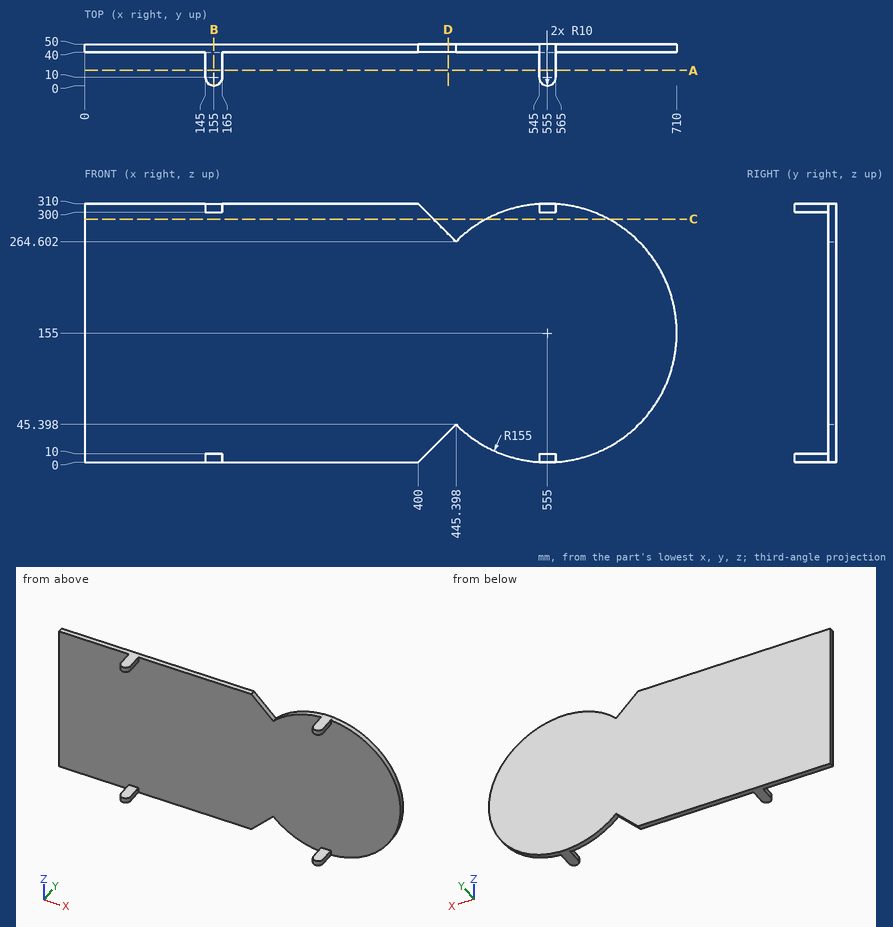
Job drawing, mm, ordinate dimensions from the low corner. One solid piece. Coordinates: 2 decimals unless noted, no trailing zeros. Order: outer loops, then holes, each group sorted by start corner. A loop starts at its lowest first (then second) coordinate and runs counter-clockwise, first axis right, second up. Notation, with made-up numbers: (24, 19) - (29, 19) arc R21 cw to (29, 24) - close; hole circle Ø4 at (31.5, 64). An arc over 180 degrees is marked (long way). Return JSON: item names as keys, results as strings. Group by question number.
1) Saw through at D-D, the plane x = 436. Write the cut outline in (y, z).
2) Probe line 1 (Y direction, x = 520, z = 125.5). List the from-to ranges inside material, lowest first. Write a range as from..to.
3) Saw through at C-C, the plane z = 291.5. Write the cut outline in (x, y) (1 decimal).
4) Saw through at B-B, the plane x = 155. Write the cut outline in (y, z), plus the area to 3 significant figures.
5) Flat gauge pins, fed straight in: P1, Ø3, axis at y = 28.5, z = 303.5, coming from the +X side; P2, Ø11, axis at y = 34, z = 306, coming from the -X side; P3, Ø1, axis at y = 38.5, z = 103.5, coming from the -X side. Where does each tip first touch, or does it go through?
6) Saw through at A-A, the plane y = 18.5. Write the cut outline in (x, z).
Values found:
{
 "1": {"outline": "(40, 36) - (50, 36) - (50, 274) - (40, 274) - close"},
 "2": {"line 1": "y = 40..50"},
 "3": {"outline": "(0, 40) - (418.5, 40) - (418.5, 50) - (0, 50) - close; (481.6, 40) - (628.4, 40) - (628.4, 50) - (481.6, 50) - close"},
 "4": {"outline": "(0, 0) - (50, 0) - (50, 310) - (0, 310) - (0, 300) - (40, 300) - (40, 10) - (0, 10) - close", "area": "3,900 mm²"},
 "5": {"P1": "stops at x = 565", "P2": "stops at x = 145", "P3": "passes through"},
 "6": {"outline": "(145, 0) - (165, 0) - (165, 10) - (145, 10) - close; (145, 300) - (165, 300) - (165, 310) - (145, 310) - close; (545, 0) - (565, 0) - (565, 10) - (545, 10) - close; (545, 300) - (565, 300) - (565, 310) - (545, 310) - close"}
}
